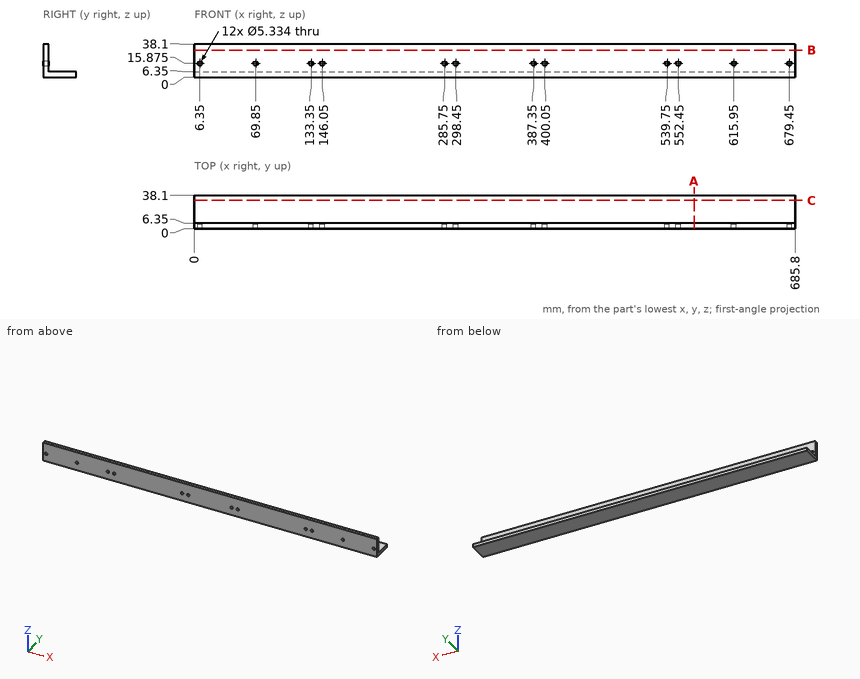
Drawing for the job (mm, zero at the part's lowest x, y, z). Give positions to 0.01 mm unless a question says otherwise; leave off trailing zeros. Order: outer loops, then holes, each group sorted by start corner. A loop starts at its lowest first (then second) coordinate and runs counter-clockwise, first axis right, second up. Notation, with made-up numbers: M 1.25,-12.5 L 48.25,-12.5 A35 cw 48.25,19.5 Z; hole C 26.25,-26.75 d9. An arc over 180 degrees is marked long. Put each result on its own line as item: value. Start each with the question number.
(1) Drill centre lines: line 1 along Z through (x, y) = (146, 2); line 2 along Y through (x, z) = (174.5, 28.5). Where is each one in solid material? Low to high.
(2) Saw through at A-A, the plane x = 570.5. Write the cut outline in (y, z).
(3) Saw through at B-B, the plane z = 31. Write the cut outline in (x, y).
(4) Flat gauge pins, fed straight in: pin 1 Ø5 at (x, z) = (6.35, 15.875) entering from -Y; pin 2 Ø6 at (x, y) = (145, 13) entering from +Z; pin 3 Ø8 at (x, z) = (470.5, 13) entering from +Y. Where does each tip first touch, or does it go through?
Check result:
1. line 1: z = 0 to 13.21, 18.54 to 38.1
1. line 2: y = 0 to 6.35
2. outline: M 0,0 L 38.1,0 L 38.1,6.35 L 6.35,6.35 L 6.35,38.1 L 0,38.1 Z
3. outline: M 0,0 L 685.8,0 L 685.8,6.35 L 0,6.35 Z
4. pin 1: passes through
4. pin 2: stops at z = 6.35
4. pin 3: stops at y = 6.35
